Here's the drawing with two shaded views (mm, measured from the low corner). I have some questions. A direction names the side the tool comes from. Give positions to 0.01 mm unless a question says otherwise; leave off trailing zeros. Write each loop counter-clockwise with the first axis right and the second up, starting at its lowest first coordinate (ties: lowest second). Pieces come first, ordered by that corner, then holes.
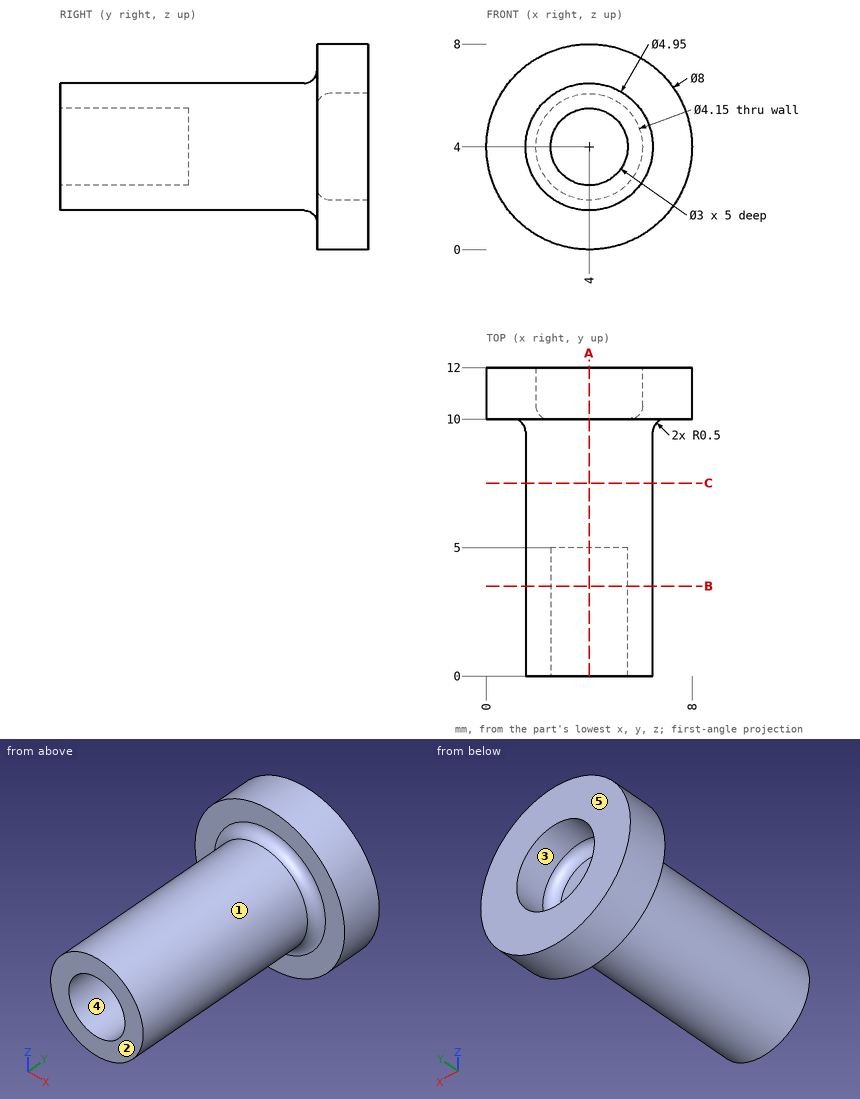
1) If we mould it in two halves opening along X, with no side actions, what happens to the marked faces 1, 2 and 3? For each: +X half, -X half, draft (parallel to the pull), parting line (faces both ways), or undercut.
Values follow:
face 1: parting line
face 2: draft
face 3: undercut
2) Suppose I cut it at C-C on y = 7.5. Write out the boundary of the cut face in (x, z) (3 decimals), plus the area to 3 significant figures.
Values follow:
outline: circle Ø4.95 at (4, 4)
area: 19.2 mm2
3) For the marked faces 4 and 5, which set-ups out of +Z, -Z, +X, -X, +Y, -Y let a thin tool reach every point of the face, with its end or its side?
Values follow:
face 4: -Y
face 5: +Z, -Z, +X, -X, +Y
4) For pin 1 Ø3 at (x, y) = (5, 7) entering from +Z (3 decimals); pin 2 Ø1.5 at (x, z) = (4, 4.5) entering from -Y; pin 3 Ø1 at (x, z) = (5, 3.5) entering from +Y, each with a flat end and sliding along its axis, tell me the tip position at first contact or that it passes through.
Values follow:
pin 1: stops at z = 6.475
pin 2: stops at y = 5
pin 3: stops at y = 10
5) Please list where these lines run through material, in increasing order: L1, parallel to Z at x = 4, y = 11.5 (3 decimals); L2, parallel to Z at x = 4, y = 1 (3 decimals).
Values follow:
L1: z = 0 to 1.925, 6.075 to 8
L2: z = 1.525 to 2.5, 5.5 to 6.475
6) Suppose I cut it at A-A on x = 4. Write out the boundary of the cut face in (y, z) (3 decimals), plus the area to 3 significant figures.
Values follow:
outline: (0, 1.525) - (9.5, 1.525) arc R0.5 cw to (10, 1.025) - (10, 0) - (12, 0) - (12, 1.925) - (10.5, 1.925) arc R0.5 cw to (10, 2.425) - (10, 5.575) arc R0.5 cw to (10.5, 6.075) - (12, 6.075) - (12, 8) - (10, 8) - (10, 6.975) arc R0.5 cw to (9.5, 6.475) - (0, 6.475) - (0, 5.5) - (5, 5.5) - (5, 2.5) - (0, 2.5) - close
area: 42.4 mm2
7) Suppose I cut it at B-B on y = 3.5. Write out the boundary of the cut face in (x, z) (3 decimals).
Values follow:
outline: circle Ø4.95 at (4, 4); hole circle Ø3 at (4, 4)
